The model under review builds one solid part; all positions refer to its coordinate system, in mm. Face numbers are marked on the shaded views. A direction names the side the tool comes from. Round coordinates to 2 decimals unless told otherwise and drop trailing zeros. Order: outer loops, then holes, each group sorted by start corner. A loop starts at its lowest first (then second) coordinate and runs counter-clockwise, first axis right, second up.
1) Consider section B-B (x = 327). Give the boundary of the cut face in (y, z), then the cut area to 3 significant figures.
2) Consider section D-D (z = 203.2). Give the number of separate pieces and of enclosed holes in the cut face, then the cut area to 3 significant figures.
3) To check wall thickness, follow L1, parallel to X at y = -74, z = 203.2; L2, parallel to X at y = -113, z = 203; L3, parallel to Z at x = 406, y = -117. State the ranges of each line that lie inside material, in increasing order.
4) Consider section C-C (z = 125). Give the boundary of the cut face in (x, y).
5) Consider section A-A (y = -114). Give the boundary of the cut face in (x, z).
6) Clearance check with flat-ended pins moving along their axes: P1, Ø1, axis at y = -98, z = 237, coming from the -X side; P2, Ø8, axis at y = -114.5, z = 237.5, coming from the +X side; P3, Ø10, axis at x = 495.5, y = -124, coming from the -Z side. State where each tip first meets the part, or that it passes through.
7) Machinability: for the marked faces 5, 6, 7, 8 and 9, which of the approach directions +Z, -Z, +X, -X, +Y, -Y give a long, thin tool a straight path to every point of the face, cutting with its end or side? Answer none if there is none.
8) Mouldability with a two-part tool opening along X and no side actions: class the marked faces 1, 2, 3 and 4 as pulls with the +X half, pulls with the -X half, needs draft (parallel to the pull), parting line crosses it, or undercut.
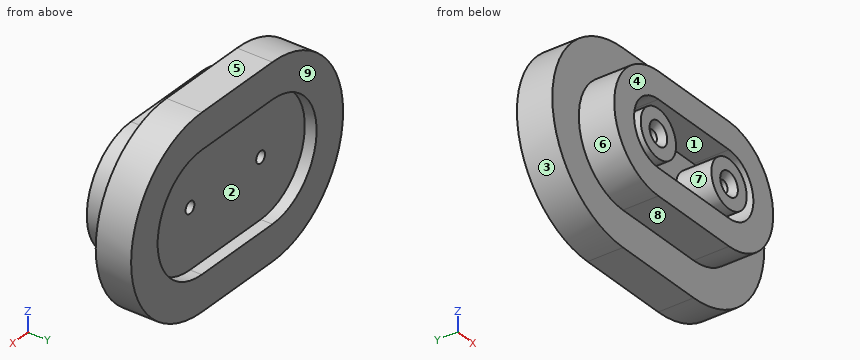
from build123d import *

# Parameters (mm, degrees)
F1_DEPTH       = 76.2
F2_START       = 25.4
F2_DEPTH       = 127
F3_START       = 25.4
F0_R           = 50.8
F3_DEPTH       = 50.8
F4_START       = 25.4
F0_R_2         = 25.4
F0_R_3         = 12.7
F4_DEPTH       = 127
F6_D           = 25.4
F6_CSINK_D     = 50.8
F6_CSINK_ANGLE = 90


with BuildPart() as f1:
    # F0 (on Front) → F1 (new body)
    with BuildSketch(Plane.XZ):
        with BuildLine():
            ThreePointArc((0, 203.2), (59.5159020629, 59.5159020629), (203.2, 0))
            Line((203.2, 0), (406.4, 0))
            ThreePointArc((406.4, 0), (550.0840979371, 59.5159020629), (609.6, 203.2))
            ThreePointArc((609.6, 203.2), (550.0840979371, 346.8840979371), (406.4, 406.4))
            Line((406.4, 406.4), (203.2, 406.4))
            ThreePointArc((203.2, 406.4), (59.5159020629, 346.8840979371), (0, 203.2))
        make_face()
        with BuildLine():
            Line((203.2, 330.2), (406.4, 330.2))
            ThreePointArc((406.4, 330.2), (533.4, 203.2), (406.4, 76.2))
            Line((406.4, 76.2), (203.2, 76.2))
            ThreePointArc((203.2, 76.2), (76.2, 203.2), (203.2, 330.2))
        make_face(mode=Mode.SUBTRACT)
    extrude(amount=F1_DEPTH)

    # F0 (on Front) → F2 (join)
    with BuildSketch(Plane.XZ.offset(F2_START)):
        with BuildLine():
            ThreePointArc((406.4, 76.2), (533.4, 203.2), (406.4, 330.2))
            Line((406.4, 330.2), (203.2, 330.2))
            ThreePointArc((203.2, 330.2), (76.2, 203.2), (203.2, 76.2))
            Line((203.2, 76.2), (406.4, 76.2))
        make_face()
        with BuildLine():
            Line((203.2, 304.8), (406.4, 304.8))
            ThreePointArc((406.4, 304.8), (508, 203.2), (406.4, 101.6))
            Line((406.4, 101.6), (203.2, 101.6))
            ThreePointArc((203.2, 101.6), (101.6, 203.2), (203.2, 304.8))
        make_face(mode=Mode.SUBTRACT)
        with BuildLine():
            ThreePointArc((406.4, 101.6), (508, 203.2), (406.4, 304.8))
            Line((406.4, 304.8), (203.2, 304.8))
            ThreePointArc((203.2, 304.8), (101.6, 203.2), (203.2, 101.6))
            Line((203.2, 101.6), (406.4, 101.6))
        make_face()
        with BuildLine():
            Line((406.4, 133.35), (203.2, 133.35))
            ThreePointArc((203.2, 133.35), (133.35, 203.2), (203.2, 273.05))
            Line((203.2, 273.05), (406.4, 273.05))
            ThreePointArc((406.4, 273.05), (476.25, 203.2), (406.4, 133.35))
        make_face(mode=Mode.SUBTRACT)
    extrude(amount=F2_DEPTH)

    # F0 (on Front) → F3 (join)
    with BuildSketch(Plane.XZ.offset(F3_START)):
        with BuildLine():
            ThreePointArc((203.2, 273.05), (133.35, 203.2), (203.2, 133.35))
            Line((203.2, 133.35), (406.4, 133.35))
            ThreePointArc((406.4, 133.35), (476.25, 203.2), (406.4, 273.05))
            Line((406.4, 273.05), (203.2, 273.05))
        make_face()
        with Locations((203.2, 203.2)):
            Circle(F0_R, mode=Mode.SUBTRACT)
        with Locations((406.4, 203.2)):
            Circle(F0_R, mode=Mode.SUBTRACT)
    extrude(amount=F3_DEPTH)

    # F0 (on Front) → F4 (join)
    with BuildSketch(Plane.XZ.offset(F4_START)):
        with Locations((406.4, 203.2)):
            Circle(F0_R)
        with Locations((406.4, 203.2)):
            Circle(F0_R_2, mode=Mode.SUBTRACT)
        with Locations((203.2, 203.2)):
            Circle(F0_R)
        with Locations((203.2, 203.2)):
            Circle(F0_R_2, mode=Mode.SUBTRACT)
        with Locations((203.2, 203.2)):
            Circle(F0_R_2)
        with Locations((203.2, 203.2)):
            Circle(F0_R_3, mode=Mode.SUBTRACT)
        with Locations((406.4, 203.2)):
            Circle(F0_R_2)
        with Locations((406.4, 203.2)):
            Circle(F0_R_3, mode=Mode.SUBTRACT)
        with Locations((203.2, 203.2)):
            Circle(F0_R_3)
        with Locations((406.4, 203.2)):
            Circle(F0_R_3)
    extrude(amount=F4_DEPTH)

    # F6 (through all)
    with Locations(Plane.XZ.offset(152.4)):
        with Locations((203.2, 203.2), (406.4, 203.2)):
            CounterSinkHole(F6_D / 2, F6_CSINK_D / 2, counter_sink_angle=F6_CSINK_ANGLE)


solid = f1.part
Answer below:
1. outline: (-152.4, 76.2) - (-76.2, 76.2) - (-76.2, 0) - (0, 0) - (0, 76.2) - (-25.4, 76.2) - (-25.4, 330.2) - (0, 330.2) - (0, 406.4) - (-76.2, 406.4) - (-76.2, 330.2) - (-152.4, 330.2) - (-152.4, 273.05) - (-76.2, 273.05) - (-76.2, 133.35) - (-152.4, 133.35) - close
1. area: 33,200 mm2
2. separate pieces: 3
2. enclosed holes: 0
2. area: 52,300 mm2
3. L1: x = 0 to 190.5, 215.9 to 393.7, 419.1 to 609.6
3. L2: x = 76.2 to 133.35, 152.4 to 190.5, 215.9 to 254, 355.6 to 393.7, 419.1 to 457.2, 476.25 to 533.4
3. L3: z = 76.2 to 133.35, 152.4 to 190.51, 215.89 to 254, 273.05 to 330.2
4. outline: (15.65, -76.2) - (103.13, -76.2) - (103.13, -152.4) - (506.47, -152.4) - (506.47, -76.2) - (593.95, -76.2) - (593.95, 0) - (506.47, 0) - (506.47, -25.4) - (103.13, -25.4) - (103.13, 0) - (15.65, 0) - close
5. outline: circle Ø101.6 at (203.2, 203.2); (203.2, 76.2) - (406.4, 76.2) arc R127 ccw to (406.4, 330.2) - (203.2, 330.2) arc R127 ccw to start; circle Ø101.6 at (406.4, 203.2); hole circle Ø25.4 at (203.2, 203.2); hole (203.2, 133.35) - (406.4, 133.35) arc R69.85 ccw to (406.4, 273.05) - (203.2, 273.05) arc R69.85 ccw to start; hole circle Ø25.4 at (406.4, 203.2)
6. P1: stops at x = 80.64
6. P2: stops at x = 529.73
6. P3: stops at z = 108.04
7. face 5: +Z, +X, -X, +Y, -Y
7. face 6: -X, -Y
7. face 7: -Y
7. face 8: -Z, +X, -X, -Y
7. face 9: +Z, -Z, +X, -X, +Y
8. face 1: undercut
8. face 2: undercut
8. face 3: pulls with the -X half
8. face 4: needs draft
